```python
from build123d import *

# Parameters (mm, degrees)
EXTRUDE_1_DEPTH = 3
SKETCH_4_R      = 0.75


with BuildPart() as part:
    # Эскиз1 → Бобышка-Вытянуть1 (new body)
    with BuildSketch(Plane.XY):
        with BuildLine():
            Line((-9, 1.5), (-6.32455532, 1.5))
            ThreePointArc((-6.32455532, 1.5), (6.5, 0), (-6.32455532, -1.5))
            Line((-6.32455532, -1.5), (-9, -1.5))
            Line((-9, -1.5), (-9, 1.5))
        make_face()
        with BuildLine():
            Line((-1.6, 0), (-1.6, 1.92045554))
            ThreePointArc((-1.6, 1.92045554), (0, 2.499629869), (1.6, 1.92045554))
            Line((1.6, 1.92045554), (1.6, -1.92045554))
            ThreePointArc((1.6, -1.92045554), (0, -2.499629869), (-1.6, -1.92045554))
            Line((-1.6, -1.92045554), (-1.6, 0))
        make_face(mode=Mode.SUBTRACT)
    extrude(amount=EXTRUDE_1_DEPTH)

    # Эскиз4 → Вырез-Повернуть1 (revolve, cut)
    with BuildSketch(Plane(origin=(0, 0, 0), x_dir=(-1, 0, 0), z_dir=(0, -1, 0))):
        with Locations((6.32455532, -1.5)):
            Circle(SKETCH_4_R)
    revolve(axis=Axis((0, 0, 0), (0, 0, -1)), mode=Mode.SUBTRACT)


solid = part.part
```
CAD build for the part. Positions are in the model's coordinates, mm. A direction names the side the tool comes from. Round coordinates to 2 decimals unless told otherwise and drop trailing zeros. Order: outer loops, then holes, each group sorted by start corner. A loop starts at its lowest first (then second) coordinate and runs counter-clockwise, first axis right, second up. Notation, with made-up numbers: (-32, 85.25) - (-9, 85.25) arc R21 cw to (-9, 96.25) - close; hole circle Ø4 at (84, 40.25). An arc over 180 degrees is marked (long way). Answer in a Markdown table with one row per item. Add a question column.
(1) Band-saw the part on A-A on y = 0. List the corners of the cut face in (x, z), and give its area (3 significant figures).
(2) Drop flat-ended pins along their axis: pin 1 Ø5 at (x, y) = (-3, 1.5) entering from -Z; pin 2 Ø1 at (x, z) = (1.5, 2.5) entering from +Y; pin 3 Ø0.8 at (x, z) = (-8, 1.5) entering from -Y; pin 4 Ø1.5 at (y, z) = (-3.5, 0.5) entering from +X. Give the stop position or say it passes through.
(3) Band-saw the part on B-B on x = 0. List the corners of the cut face in (y, z), and give its area (3 significant figures).
(4) 3-axis set-ups, long thin cutter, end or side, ignore diameter. For faces 4 (the face through (-8, 1.5, 1)), 5 (the face through (-3, 0, 0)), 6 (the face through (-1.6, 0, 1)): which of +Z, -Z, +X, -X, +Y, -Y reach the whole face in a straight line?
(5) Band-saw the part on C-C on z = 2.65. List the corners of the cut face in (x, y).
(6) Mould opens along X. For faces 1 (the face through (6.495, 0.265, 2.609)), 2 (the face through (0, -2.5, 1.5)), 3 (the face through (-8, -1.5, 1)) say: +X half, -X half, draft (parallel to the pull), parting line (faces both ways), or undercut.
(7) Probe L1, parallel to X at y = 1, z = 1.15; L2, parallel to X at y = -0.25, z = 1.05; L3, parallel to Z at x = -5.25, y = 2.25. List the from-to ranges inside material, lowest first. Write a range as [from, to].
Data:
| question | item | result |
|---|---|---|
| 1 | outline | (-9, 0) - (-1.6, 0) - (-1.6, 3) - (-9, 3) - close; (1.6, 0) - (6.5, 0) - (6.5, 0.77) arc R0.75 cw (long way) to (6.5, 2.23) - (6.5, 3) - (1.6, 3) - close; hole circle Ø1.5 at (-6.32, 1.5) |
| 1 | area | 34.0 mm^2 |
| 2 | pin 1 | stops at z = 0 |
| 2 | pin 2 | stops at y = 6.42 |
| 2 | pin 3 | stops at y = -1.5 |
| 2 | pin 4 | stops at x = 5.89 |
| 3 | outline | (-6.5, 0) - (-2.5, 0) - (-2.5, 3) - (-6.5, 3) - (-6.5, 2.23) arc R0.75 cw (long way) to (-6.5, 0.77) - close; (2.5, 0) - (6.5, 0) - (6.5, 0.77) arc R0.75 cw (long way) to (6.5, 2.23) - (6.5, 3) - (2.5, 3) - close |
| 3 | area | 21.7 mm^2 |
| 4 | face 4 | +Z, -Z, -X, +Y |
| 4 | face 5 | -Z, +X, -X, +Y, -Y |
| 4 | face 6 | +Z, -Z |
| 5 | outline | (-9, -1.5) - (-6.32, -1.5) arc R6.5 ccw (long way) to (-6.32, 1.5) - (-9, 1.5) - close; hole (-1.6, -1.92) arc R2.5 ccw to (1.6, -1.92) - (1.6, 1.92) arc R2.5 ccw to (-1.6, 1.92) - close |
| 6 | face 1 | parting line |
| 6 | face 2 | undercut |
| 6 | face 3 | draft |
| 7 | L1 | x = [-9, -6.92], [-5.57, -1.6], [1.6, 5.57] |
| 7 | L2 | x = [-9, -6.92], [-5.72, -1.6], [1.6, 5.72] |
| 7 | L3 | z = [0, 1.07], [1.93, 3] |
